Verification items for the finished model (mm, model axes). Give positions to 0.01 mm unless a question says otherwise; leave off trailing zeros. Answer in a Markdown table with one row per item.
```python
from build123d import *

# Parameters (mm, degrees)
F0_W     = 30
F0_H     = 6
F1_DEPTH = 200
F2_R     = 0.8
F2_R_2   = 4
F3_DEPTH = 6


with BuildPart() as f1:
    # F0 (on Top) → F1 (new body, symmetric)
    with BuildSketch(Plane.XY):
        Rectangle(F0_W, F0_H)
    extrude(amount=F1_DEPTH, both=True)

    # F2 (on face) → F3 (cut, through all)
    with BuildSketch(Plane.XZ.offset(3)):
        with Locations((0, 196.2)):
            Circle(F2_R)
        with Locations((0, 188.2)):
            Circle(F2_R_2)
        with Locations((-5.656854, 193.856854)):
            Circle(F2_R)
        with Locations((-8, 188.2)):
            Circle(F2_R)
        with Locations((-5.656854, 182.543146)):
            Circle(F2_R)
        with Locations((0, 180.2)):
            Circle(F2_R)
        with Locations((5.656854, 182.543146)):
            Circle(F2_R)
        with Locations((8, 188.2)):
            Circle(F2_R)
        with Locations((5.656854, 193.856854)):
            Circle(F2_R)
    extrude(amount=-F3_DEPTH, mode=Mode.SUBTRACT)


solid = f1.part
```
Q1. Go/stop test with a flat-tipped pin: P1, Ø1.3, axis at x = 8, z = 188.2, coming from the -Y side. Record where the tip stops, or that it passes through.
Completed:
| item | result |
|---|---|
| P1 | through |
Q2. Thickness scan on line 1 (Z direction, x = 0, y = 0.7); line 2 (Z direction, x = -5.5, y = -1.1); line 3 (X direction, y = 0.7, z = 180.2). Record the ranges inside material, lowest first.
Completed:
| item | result |
|---|---|
| line 1 | -200 to 179.4, 181 to 184.2, 192.2 to 195.4, 197 to 200 |
| line 2 | -200 to 181.76, 183.33 to 193.07, 194.64 to 200 |
| line 3 | -15 to -0.8, 0.8 to 15 |
Q3. Draft check along Z on faces 1 (the face through (-0.867, -0.042, 184.295)), 2 (the face through (0, 3, 3)). Enter one of: +Z half, -Z half, draft (parallel to the pull), parting line (faces both ways), or undercut.
Completed:
| item | result |
|---|---|
| face 1 | undercut |
| face 2 | draft |
